Part model, mm, in its own coordinate system. Face numbers are marked on the shaded views. A direction names the side the tool comes from. Give positions to 0.01 mm unless a question says otherwise; leave off trailing zeros. Write each loop counter-clockwise with the first axis right and the second up, starting at its lowest first coordinate (ties: lowest second). Pieces come first, ordered by that corner, then holes. Notation, with made-up numbers: M 34.25,14 L 83.25,14 A18 cw 83.25,18 Z; hole C 41.25,-38.5 d4. An arc over 180 degrees is marked long. Answer as CSV lines item,"result". Start each with the question number.
1) Tool access for the marked faces 4, 5, 6, 7 and 8: list every direction of +Z, -Z, +X, -X, +Y, -Y with a clear straight run to the whole face (end or side of a thin tool).
2) Mould opens along Z. For the marked faces 1, 2 and 3 say: pulls with the +Z half, pulls with the -Z half, needs draft (parallel to the pull), parting line crosses it, or undercut.
3) Slice it at A-A, the plane x = 0. Give the number of separate pieces and of enclosed holes in the cut face, plus the area to 3 significant figures.
4) Pin check, flat tips, straight feed: pin 1 Ø2.5 at (x, y) = (1, -9.5) entering from -Z; pin 2 Ø1.6 at (x, y) = (-3, -19.13) entering from -Z; pin 3 Ø2.5 at (x, y) = (0, -19.47) entering from +Z. Stop position of each tip, or through.
5) Wall check: line 1 along Y through (x, z) = (-3, 9.15); line 2 along Z through (x, y) = (-3, 0.5); line 3 along Z through (x, y) = (-3.75, 4.25). Give the ranges that are in metal, low to high. Write a range as from..to.
6) Slice it at B-B, the plane y = -15.5. Give the cut face in (x, z), plus the area to 3 significant figures.
7) Slice it at C-C, the plane z = 4. Give the cut face in (x, y).
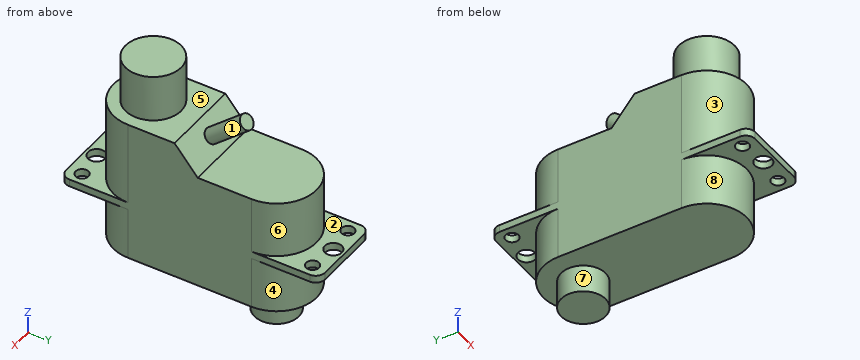
```python
from build123d import *

# Parameters (mm, degrees)
SKETCH1_R               = 2.4
BOSS_EXTRUDE1_DEPTH     = 3
BOSS_EXTRUDE2_DEPTH     = 15.51
CUT_EXTRUDE1_DEPTH      = 5.31
CUT_EXTRUDE1_DEPTH_BACK = 5.31
SKETCH4_R               = 3.01
BOSS_EXTRUDE3_DEPTH     = 5.06
SKETCH5_R               = 0.925
SKETCH5_R_2             = 0.7
BOSS_EXTRUDE4_DEPTH     = 0.8
SKETCH6_R               = 0.823117729
BOSS_EXTRUDE5_DEPTH     = 5


with BuildPart() as part:
    # Sketch1 → Boss-Extrude1 (new body)
    with BuildSketch(Plane.XY):
        Circle(SKETCH1_R)
    extrude(amount=BOSS_EXTRUDE1_DEPTH)

    # Sketch2 → Boss-Extrude2 (add)
    with BuildSketch(Plane.XY.offset(3)):
        with BuildLine():
            Line((4.31, 0), (4.31, -13.34))
            ThreePointArc((4.31, -13.34), (0, -17.65), (-4.31, -13.34))
            Line((-4.31, -13.34), (-4.31, 0))
            ThreePointArc((-4.31, 0), (0, 4.31), (4.31, 0))
        make_face()
    extrude(amount=BOSS_EXTRUDE2_DEPTH)

    # Sketch3 → Cut-Extrude1 (cut, two sides)
    with BuildSketch(Plane(origin=(0, 0, 0), x_dir=(0, 0, -1), z_dir=(1, 0, 0))) as cut_extrude1_sk:
        Polygon((-18.51, 4.31), (-15.55, 4.31), (-15.55, -5.79), (-18.51, -8.3), align=None)
    extrude(amount=CUT_EXTRUDE1_DEPTH, mode=Mode.SUBTRACT)
    extrude(cut_extrude1_sk.sketch, amount=-CUT_EXTRUDE1_DEPTH_BACK, mode=Mode.SUBTRACT)

    # Sketch4 → Boss-Extrude3 (add)
    with BuildSketch(Plane.XY.offset(18.51)):
        with Locations((0, -13.34)):
            Circle(SKETCH4_R)
    extrude(amount=BOSS_EXTRUDE3_DEPTH)

    # Sketch5 → Boss-Extrude4 (add)
    with BuildSketch(Plane(origin=(0, 0, 8.63), x_dir=(-1, 0, 0), z_dir=(0, 0, -1))):
        with BuildLine():
            Line((-3.31, 7.33), (3.31, 7.33))
            ThreePointArc((3.31, 7.33), (4.017106781, 7.037106781), (4.31, 6.33))
            Line((4.31, 6.33), (4.31, -19.67))
            ThreePointArc((4.31, -19.67), (4.017106781, -20.377106781), (3.31, -20.67))
            Line((3.31, -20.67), (-3.31, -20.67))
            ThreePointArc((-3.31, -20.67), (-4.017106781, -20.377106781), (-4.31, -19.67))
            Line((-4.31, -19.67), (-4.31, 6.33))
            ThreePointArc((-4.31, 6.33), (-4.017106781, 7.037106781), (-3.31, 7.33))
        make_face()
        with Locations((0, 6.13)):
            Circle(SKETCH5_R, mode=Mode.SUBTRACT)
        with Locations((3, 5.79076381)):
            Circle(SKETCH5_R_2, mode=Mode.SUBTRACT)
        with Locations((-3, 5.79076381)):
            Circle(SKETCH5_R_2, mode=Mode.SUBTRACT)
        with Locations((3, -19.13076381)):
            Circle(SKETCH5_R_2, mode=Mode.SUBTRACT)
        with Locations((0, -19.47)):
            Circle(SKETCH5_R, mode=Mode.SUBTRACT)
        with Locations((-3, -19.13076381)):
            Circle(SKETCH5_R_2, mode=Mode.SUBTRACT)
    extrude(amount=-BOSS_EXTRUDE4_DEPTH)

    # Sketch6 → Boss-Extrude5 (add)
    with BuildSketch(Plane(origin=(0, 4.302344091, 3.64827151), x_dir=(1, 0, 0), z_dir=(0, 0.7627017, 0.646750428))):
        with Locations((0, -17.550441075)):
            Circle(SKETCH6_R)
    extrude(amount=BOSS_EXTRUDE5_DEPTH)


solid = part.part
```
Found:
1,face 4,"-Z, +Y"
1,face 5,"+Z"
1,face 6,"+Z, +Y"
1,face 7,"-Z"
1,face 8,"-Z, -Y"
2,face 1,"undercut"
2,face 2,"pulls with the +Z half"
2,face 3,"needs draft"
3,separate pieces,"3"
3,enclosed holes,"0"
3,area,"362 mm²"
4,pin 1,"z = 3"
4,pin 2,"z = 8.63"
4,pin 3,"z = 9.43"
5,line 1,"-20.67..-19.83, -18.43..5.09, 6.49..7.33"
5,line 2,"3..15.55"
5,line 3,"8.63..9.43"
6,outline,"M -4.31,8.63 L -3.73,8.63 L -3.73,3 L 3.73,3 L 3.73,8.63 L 4.31,8.63 L 4.31,9.43 L 3.73,9.43 L 3.73,18.51 L 2.1,18.51 L 2.1,23.57 L -2.1,23.57 L -2.1,18.51 L -3.73,18.51 L -3.73,9.43 L -4.31,9.43 Z"
6,area,"138 mm²"
7,outline,"M -4.31,-13.34 A4.31 ccw 4.31,-13.34 L 4.31,0 A4.31 ccw -4.31,0 Z"
